The figure shows three views and two pictorial views of one solid part (mm, origin at its lowest corner). Answer the questions. A direction names the side the tool comes from. Give positions to 0.01 mm unless a question says otherwise; leave off trailing zeros. Loops run counter-clockwise (first coordinate to the right, second up) from the corner with the lowest first, then second, coordinate; pieces in that order, holes last. Notation, with made-up numbers: (65.25, 29) - (117.25, 29) arc R11 ccw to (117.25, 34) - close; hole circle Ø8 at (74.5, -22.5). An arc over 180 degrees is marked (long way). Use a Markdown table: item, result. Add a question column.
Item 1: Each of these flat-tipped pins is pushed along its axis until it touches: P1, Ø4, axis at x = 22, z = 1.5, coming from the -Y side; P2, Ø1.6, axis at y = 22.5, z = 3.5, coming from the -X side; P3, Ø2, axis at x = 6.5, y = 23, coming from the +Z side; P4, Ø2, axis at x = 9.5, y = 17.5, coming from the -Z side. Where does it stop, or does it pass through?
Item 2: A cutting plane is placed at A-A (y = 18). Determine the outline of the cut face in (x, z), plus the area to 3 significant figures.
Item 3: A cutting plane is placed at B-B (z = 3.5). Give the number of separate pieces and of enclosed holes in the cut face, plus the area to 3 significant figures.
Item 4: A cutting plane is placed at C-C (x = 17.25). Determine the outline of the cut face in (y, z).
Item 5: Consider probe 1 along Y at (x, z) = (16.15, 3.5); probe 2 along X at (y, z) = (2, 0.5); probe 3 along X at (y, z) = (27, 4.5). Determine where each line is inside the solid, lowest interval first. Write a range as [from, to].
Item 6: Which of the six approach directions +Z, -Z, +X, -X, +Y, -Y give full straight-line access (tool end or side, diameter ignored) to the marked faces 1, 2, 3, 4 and 5?
Item 7: For a pull along Y with two mould halves and no side action, classify the marked faces 6, 7 and 8 as +Y half, -Y half, draft (parallel to the pull), parting line (faces both ways), or undercut.
Item 8: A cutting plane is placed at D-D (y = 13.5). Determine the outline of the cut face in (x, z), plus the area to 3 significant figures.
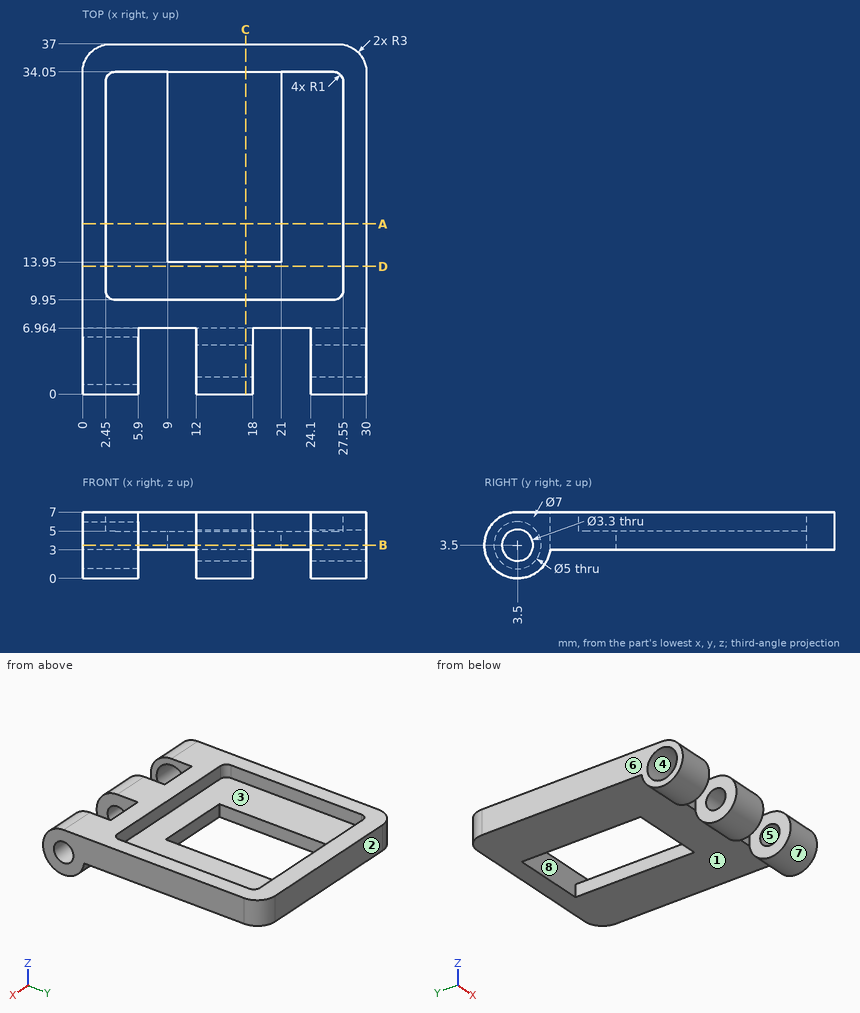
Geometry says:
| question | item | result |
|---|---|---|
| 1 | P1 | y = 6.96 |
| 1 | P2 | x = 0 |
| 1 | P3 | z = 5 |
| 1 | P4 | z = 3 |
| 2 | outline | (0, 3) - (9, 3) - (9, 5) - (2.45, 5) - (2.45, 7) - (0, 7) - close; (21, 3) - (30, 3) - (30, 7) - (27.55, 7) - (27.55, 5) - (21, 5) - close |
| 2 | area | 45.8 mm² |
| 3 | separate pieces | 4 |
| 3 | enclosed holes | 1 |
| 3 | area | 711 mm² |
| 4 | outline | (3.5, 7) arc R3.5 ccw (long way) to (6.96, 3) - (13.95, 3) - (13.95, 5) - (9.95, 5) - (9.95, 7) - close; (34.05, 3) - (37, 3) - (37, 7) - (34.05, 7) - close; hole circle Ø3.3 at (3.5, 3.5) |
| 5 | probe 1 | [0, 1.85], [5.15, 13.95], [34.05, 37] |
| 5 | probe 2 | [0, 5.9], [12, 18], [24.1, 30] |
| 5 | probe 3 | [0, 9], [21, 30] |
| 6 | face 1 | -Z, +X, -X, +Y |
| 6 | face 2 | +Z, -Z, +X, -X, +Y |
| 6 | face 3 | +Z |
| 6 | face 4 | -X |
| 6 | face 5 | +X, -X |
| 7 | face 6 | draft |
| 7 | face 7 | parting line |
| 7 | face 8 | undercut |
| 8 | outline | (0, 3) - (30, 3) - (30, 7) - (27.55, 7) - (27.55, 5) - (2.45, 5) - (2.45, 7) - (0, 7) - close |
| 8 | area | 69.8 mm² |
